```python
from build123d import *

# Parameters (mm, degrees)
SKETCH1_W             = 44
SKETCH1_H             = 20
JOINER_PLATE_DEPTH    = 3
BOLT_HOLES_DEPTH      = 25.351591324
BOLT_HOLES_DEPTH_BACK = 25.351591324
SKETCH2_R             = 1.7


with BuildPart() as part:
    # Sketch1 → Joiner Plate (new body)
    with BuildSketch(Plane(origin=(0, 0, 0), x_dir=(1, 0, 0), z_dir=(0, 1, 0))):
        Rectangle(SKETCH1_W, SKETCH1_H)
    extrude(amount=JOINER_PLATE_DEPTH)

    # Sketch2 → Bolt Holes (cut, two sides: drawn at the far end of the back side and taken through both)
    with BuildSketch(Plane(origin=(0, 0, 0), x_dir=(1, 0, 0), z_dir=(0, 1, 0)).offset(-BOLT_HOLES_DEPTH_BACK)):
        with Locations(Location((-12, 0, 0), (0, 0, 270))):
            Circle(SKETCH2_R)
        with Locations(Location((12, 0, 0), (0, 0, 270))):
            Circle(SKETCH2_R)
    extrude(amount=BOLT_HOLES_DEPTH + BOLT_HOLES_DEPTH_BACK, mode=Mode.SUBTRACT)


solid = part.part
```
Read the model definition and answer for the solid it produces. Units are mm, in the model's axes. Give positions to 0.01 mm unless a question says otherwise; leave off trailing zeros. Order: outer loops, then holes, each group sorted by start corner. A loop starts at its lowest first (then second) coordinate and runs counter-clockwise, first axis right, second up.
(1) Find section C-C (y = 2.55). Give the vertices of the cut face in (x, z).
(2) For a pull along Z with two mould halves and no side action, classify faces 1 (the flat face through (0, 0, 0)), 2 (the flat face through (0, 1, -10)), 3 (the flat face through (0, 1, 10)), 4 (the cylindrical face through (13.686, 1.479, -0.221)) as released by +Z, released by -Z, zero draft, split by the parting line, or undercut.
(3) Find section D-D (x = 13). Give the vertices of the cut face in (y, z), plus the area to 3 significant figures.
(4) Straight lines are drawn through the part: L1, parallel to X at y = 2.25, z = 0; L2, parallel to Z at x = -12, y = 2.4; L3, parallel to X at y = 2.75, z = -1.25. For each, find the intervals that lie inside material, in ascending order.
(5) Find section B-B (x = -12). Give the vertices of the cut face in (y, z), plus the area to 3 significant figures.
(6) Find section A-A (z = 0). Give the vertices of the cut face in (x, y), plus the area to 3 significant figures.
Result sheet:
1. outline: (-22, -10) - (22, -10) - (22, 10) - (-22, 10) - close; hole circle Ø3.4 at (-12, 0); hole circle Ø3.4 at (12, 0)
2. face 1: zero draft
2. face 2: released by -Z
2. face 3: released by +Z
2. face 4: undercut
3. outline: (0, -10) - (3, -10) - (3, -1.37) - (0, -1.37) - close; (0, 1.37) - (3, 1.37) - (3, 10) - (0, 10) - close
3. area: 51.8 mm2
4. L1: x = -22 to -13.7, -10.3 to 10.3, 13.7 to 22
4. L2: z = -10 to -1.7, 1.7 to 10
4. L3: x = -22 to -13.15, -10.85 to 10.85, 13.15 to 22
5. outline: (0, -10) - (3, -10) - (3, -1.7) - (0, -1.7) - close; (0, 1.7) - (3, 1.7) - (3, 10) - (0, 10) - close
5. area: 49.8 mm2
6. outline: (-22, 0) - (-13.7, 0) - (-13.7, 3) - (-22, 3) - close; (-10.3, 0) - (10.3, 0) - (10.3, 3) - (-10.3, 3) - close; (13.7, 0) - (22, 0) - (22, 3) - (13.7, 3) - close
6. area: 112 mm2
